Build history of the part. All positions in model axes, mm. A direction names the side the tool comes from. Round coordinates to 2 decimals unless told otherwise and drop trailing zeros. Loops run counter-clockwise (first coordinate to the right, second up) from the corner with the lowest first, then second, coordinate; pieces in that order, holes last. Notation, with made-up numbers: (-6.5, 45) - (19.5, 45) arc R33 ccw to (19.5, 84) - close; hole circle Ø10 at (31, -14). An arc over 180 degrees is marked (long way). Answer as CSV lines item,"result". Start each with the question number.
Autodesk Inventor part; units mm, degrees
ref_plane "YZ Plane" through (0, 0, 0) normal (1, 0, 0) x (0, 1, 0)
ref_plane "XZ Plane" through (0, 0, 0) normal (0, 1, 0) x (-1, 0, 0)
ref_plane "XY Plane" through (0, 0, 0) normal (0, 0, 1) x (1, 0, 0)
sketch "Sketch2" plane through (0, 0, 0) normal (0, 1, 0) x (-1, 0, 0)
  line L0 (0, 0) -> (0, 127)
  line L1 (0, 127) -> (127, 127)
  line L2 (127, 127) -> (127, 0)
  line L3 (127, 0) -> (0, 0)
  arc A0 (9.525, 107.95) -> (9.525, 101.6) centre (9.525, 104.775) ccw
  arc A1 (47.625, 101.6) -> (47.625, 107.95) centre (47.625, 104.775) ccw
  arc A2 (47.625, 73.025) -> (47.625, 79.375) centre (47.625, 76.2) ccw
  arc A3 (9.525, 79.375) -> (9.525, 73.025) centre (9.525, 76.2) ccw
  line L4 (9.525, 79.375) -> (47.625, 79.375)
  line L5 (47.625, 73.025) -> (9.525, 73.025)
  line L6 (9.525, 107.95) -> (47.625, 107.95)
  line L7 (47.625, 101.6) -> (9.525, 101.6)
  line L8 (9.525, 104.775) -> (9.525, 76.2) construction
  circle A4 centre (114.3, 114.3) radius 3.175
  circle A5 centre (114.3, 38.1) radius 3.175
  circle A6 centre (12.7, 12.7) radius 3.175
  circle A7 centre (88.9, 12.7) radius 3.175
  line L9 (114.3, 114.3) -> (114.3, 38.1) construction
  line L10 (12.7, 12.7) -> (88.9, 12.7) construction
  dimension "d7" = 127
  dimension "d18" = 38.1
  dimension "d19" = 79.375
  dimension "d22" = 12.7
  dimension "d23" = 76.2
  dimension "d24" = 76.2
  dimension "d25" = 6.35
  dimension "d28" = 12.7
  dimension "d29" = 12.7
  dimension "d30" = 38.1
  dimension "d31" = 127
  dimension "d32" = 9.525
  dimension "d36" = 12.7
  dimension "d39" = 22.225
  dimension "d40" = 28.575
  dimension "d41" = 76.2
extrude "Extrusion3" add sketch "Sketch2" along normal blind 3.175
chamfer "Chamfer1" distance 25.4 angle 45 1 edges at (-127, 1.5875, 0)
properties part number "GearboxMountPlate" material "Aluminum-6061"
Q1. Tool access for faces 5 (the flat face through (-28, 2, 107.95)), 6 (the flat face through (-63, 0, 64)): list every direction of +Z, -Z, +X, -X, +Y, -Y with a clear straight run to the whole face (end or side of a thin tool).
Q2. Band-saw the part on A-A, the plane z = 38.1. List the corners of the cut face in (x, y) (3 decimals), then the cut area to 3 significant figures.
Q3. Pin check, flat tip, straight feed: pin 1 Ø4 at (x, z) = (-85.5, 96.5) entering from -Y. Stop position of the tip, or through.
Q4. Band-saw the part on D-D, the plane x = -88.9. List the corners of the cut face in (y, z) (3 decimals), then the cut area to 3 significant figures.
Q5. Wall check: probe 1 along Z at (x, y) = (-31, 1.4) (3 decimals); probe 2 along Z at (x, y) = (-12.7, 2.2) (3 decimals); probe 3 along Z at (x, y) = (-114.3, 2.25) (3 decimals). Give the ranges that are in metal, low to high. Write a range as [from, to].
Q6. Band-saw the part on C-C, the plane z = 12.7. List the corners of the cut face in (x, y) (3 decimals).
Q7. Band-saw the part on B-B, the plane x = -12.7. List the corners of the cut face in (y, z) (3 decimals).
Q8. Two-plate mould, pull along X, no slides. Class faces 1 (the flat face through (0, 2, 63)), 2 (the cylindrical face through (-116.007, 1.565, 35.423)), 3 (the flat face through (-52, 2, 0)), 4 (the flat face through (-114.1, 1.6, 12.5)): released by +X, released by -X, zero draft, split by the parting line, or undercut.
Reported:
1,face 5,"+Y, -Y"
1,face 6,"+Z, -Z, +X, -X, -Y"
2,outline,"(-127, 0) - (-117.475, 0) - (-117.475, 3.175) - (-127, 3.175) - close; (-111.125, 0) - (0, 0) - (0, 3.175) - (-111.125, 3.175) - close"
2,area,"383 mm2"
3,pin 1,"stops at y = 0"
4,outline,"(0, 0) - (3.175, 0) - (3.175, 9.525) - (0, 9.525) - close; (0, 15.875) - (3.175, 15.875) - (3.175, 127) - (0, 127) - close"
4,area,"383 mm2"
5,probe 1,"z = [0, 73.025], [79.375, 101.6], [107.95, 127]"
5,probe 2,"z = [0, 9.525], [15.875, 73.025], [79.375, 101.6], [107.95, 127]"
5,probe 3,"z = [12.7, 34.925], [41.275, 111.125], [117.475, 127]"
6,outline,"(-114.3, 0) - (-92.075, 0) - (-92.075, 3.175) - (-114.3, 3.175) - close; (-85.725, 0) - (-15.875, 0) - (-15.875, 3.175) - (-85.725, 3.175) - close; (-9.525, 0) - (0, 0) - (0, 3.175) - (-9.525, 3.175) - close"
7,outline,"(0, 0) - (3.175, 0) - (3.175, 9.525) - (0, 9.525) - close; (0, 15.875) - (3.175, 15.875) - (3.175, 73.025) - (0, 73.025) - close; (0, 79.375) - (3.175, 79.375) - (3.175, 101.6) - (0, 101.6) - close; (0, 107.95) - (3.175, 107.95) - (3.175, 127) - (0, 127) - close"
8,face 1,"released by +X"
8,face 2,"undercut"
8,face 3,"zero draft"
8,face 4,"released by -X"
